Part model, mm, in its own coordinate system. Face numbers are marked on the shaded views. Round coordinates to 2 decimals unless told otherwise and drop trailing zeros. Write each loop counter-clockwise with the first axis right and the second up, starting at its lowest first coordinate (ties: lowest second). Pieces come first, ordered by that corner, then holes. Notation, with made-up numbers: (8, 14.25) -> (49, 14.25) arc R33 ccw to (49, 51.25) -> close; hole circle Ø1 at (78.25, 6.25). An arc over 180 degrees is marked (long way). Return JSON: item names as keys, results as strings. Group by question number.
(1) Saw through at C-C (x = -34). List the corners of the cut face in (y, z).
(2) Saw through at D-D (x = 174). List the corners of the cut face in (y, z).
(3) Drop flat-ended pins along their axis: pin 1 Ø12 at (x, y) = (-64.5, -77) entering from +Z; pin 2 Ø6.5 at (y, z) = (13, 6) entering from -X; pin 3 Ø15 at (y, z) = (-72.5, 26.5) entering from -X. Give the stop position or say it passes through.
(4) Mould opens along Y. For the marked faces 1, 2, 3 and 4 say: +Y half, -Y half, draft (parallel to the pull), parting line (faces both ways), or undercut.
(5) Saw through at A-A (z = 35). List the corners of the cut face in (x, y), plus the area to 3 significant figures.
(6) Drill centre lines: L1, parallel to Y at x = -13, z = 19.5; L2, parallel to X at y = 4.5, z = 13; L3, parallel to Z at x = 172.5, y = 88.5. Where is each one in solid material? Low to high. Write a range as from..to.
(7) Saw through at B-B (y = 93). List the corners of the cut face in (x, z), plus the area to 3 significant figures.
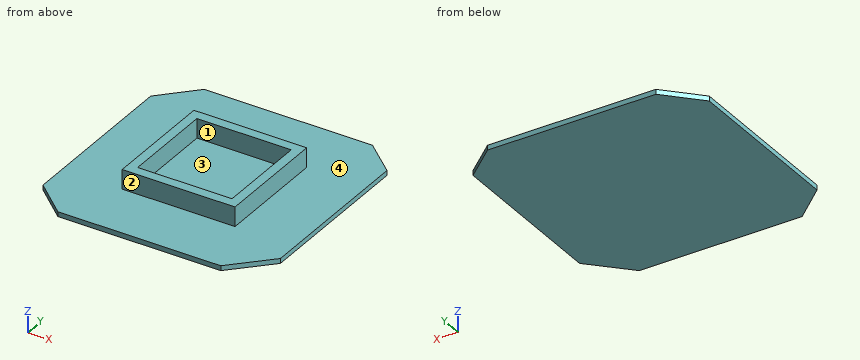
from build123d import *

# Parameters (mm, degrees)
F1_DEPTH = 12.7
F3_W     = 295.542716
F3_H     = 296.202182
F3_W_2   = 246.921896
F3_H_2   = 244.63451
F4_DEPTH = 50.8


with BuildPart() as f1:
    # F0 (on Top) → F1 (new body)
    with BuildSketch(Plane.XY):
        Polygon((304.8, 231.870204), (220.464751, 304.8), (-220.213354, 304.8), (-304.8, 217.583231), (-304.8, 217.559303), (-304.8, -227.374971), (-216.906339, -304.8), (209.789738, -304.8), (304.8, -208.257139), align=None)
        Polygon((-304.8, 217.559303), (-304.8, 217.583231), (-304.983646, 217.393875), align=None)
    extrude(amount=F1_DEPTH)

    # F3 (on face) → F4 (join)
    with BuildSketch(Plane.XY.offset(12.7)):
        Rectangle(F3_W, F3_H)
        Rectangle(F3_W_2, F3_H_2, mode=Mode.SUBTRACT)
    extrude(amount=F4_DEPTH)


solid = f1.part
Computed values:
{
 "1": {"outline": "(-304.8, 0) -> (304.8, 0) -> (304.8, 12.7) -> (148.1, 12.7) -> (148.1, 63.5) -> (122.32, 63.5) -> (122.32, 12.7) -> (-122.32, 12.7) -> (-122.32, 63.5) -> (-148.1, 63.5) -> (-148.1, 12.7) -> (-304.8, 12.7) -> close"},
 "2": {"outline": "(-304.8, 0) -> (304.8, 0) -> (304.8, 12.7) -> (-304.8, 12.7) -> close"},
 "3": {"pin 1": "z = 12.7", "pin 2": "x = -304.8", "pin 3": "x = -147.77"},
 "4": {"face 1": "undercut", "face 2": "-Y half", "face 3": "undercut", "face 4": "draft"},
 "5": {"outline": "(-147.77, -148.1) -> (147.77, -148.1) -> (147.77, 148.1) -> (-147.77, 148.1) -> close; hole (-123.46, -122.32) -> (123.46, -122.32) -> (123.46, 122.32) -> (-123.46, 122.32) -> close", "area": "27,100 mm2"},
 "6": {"L1": "-148.1..-122.32, 122.32..148.1", "L2": "-147.77..-123.46, 123.46..147.77", "L3": "0..12.7"},
 "7": {"outline": "(-304.8, 0) -> (304.8, 0) -> (304.8, 12.7) -> (147.77, 12.7) -> (147.77, 63.5) -> (123.46, 63.5) -> (123.46, 12.7) -> (-123.46, 12.7) -> (-123.46, 63.5) -> (-147.77, 63.5) -> (-147.77, 12.7) -> (-304.8, 12.7) -> close", "area": "10,200 mm2"}
}
